The model under review builds one solid part; all positions refer to its coordinate system, in mm. Face numbers are marked on the shaded views. A direction names the side the tool comes from. Round coordinates to 2 decimals unless told otherwise and drop trailing zeros. Order: outer loops, then holes, each group sorted by start corner. A loop starts at its lowest first (then second) coordinate and runs counter-clockwise, first axis right, second up. Notation, with made-up numbers: M -26,72 L 10,72 A21 ccw 10,76 Z; hole C 76.5,56 d5. An arc over 180 degrees is marked long. Answer as a JSON object with one key per item and string values. Group by question number.
1. Add section C-C on y = 0.25. State the section outline as (x, z) points.
2. Add section A-A on z = 4.5. State the section outline as (x, y) points.
3. To check wall thickness, follow probe 1 along Y at (x, z) = (-1, -2.5); probe 2 along Y at (x, z) = (-1.5, 6.5); probe 3 along Z at (x, y) = (-2.25, 3). State the ranges of each line that lie inside material, in increasing order. Write a range as [from, to].
4. Add section D-D on z = -5.75. State the section outline as (x, y) points, and give its area (4 significant figures).
5. Mouldability with a two-part tool opening along Y and no side actions: class the marked faces 1, 2, 3 and 4 as released by +Y, released by -Y, zero draft, split by the parting line, or undercut.
6. Clearance check with flat-ended pins moving along their axes: P1, Ø0.5, axis at y = -0.5, z = -4.5, coming from the +X side; P2, Ø3, axis at x = 0, z = 0, coming from the +Y side. State where each tip first meets the part, or that it passes through.
7. Machinability: for the marked faces 5 and 6, which of the approach directions +Z, -Z, +X, -X, +Y, -Y give a long, thin tool a straight path to every point of the face, cutting with its end or side? Answer none if there is none.
8. Add section B-B on x = -0.25. State the section outline as (y, z) points, and give its area (3 significant figures).
Autodesk Inventor part; units mm, degrees
ref_plane "YZ Plane" through (0, 0, 0) normal (1, 0, 0) x (0, 1, 0)
ref_plane "XZ Plane" through (0, 0, 0) normal (0, 1, 0) x (-1, 0, 0)
ref_plane "XY Plane" through (0, 0, 0) normal (0, 0, 1) x (1, 0, 0)
sketch "スケッチ1" plane through (0, 0, 0) normal (0, 1, 0) x (-1, 0, 0)
  circle A0 centre (0, 0) radius 1.15
  circle A1 centre (0, 0) radius 2
  circle A2 centre (0, 0) radius 3.5
  line L0 (0, 0) -> (0, 3.5)
  line L1 (2, 0) -> (-2, 0)
  line L2 (2, 0) -> (2, -2.8723)
  line L3 (-2, 0) -> (-2, -2.8723)
  line L4 (0, 2) -> (3.5, 2)
  line L5 (3.5, 2) -> (3.5, 6)
  line L6 (3.5, 6) -> (0, 6)
  line L7 (0, 6) -> (0, 2)
  line L8 (0, 6) -> (3.5, 6)
  line L9 (3.5, 6) -> (3.5, 0)
  line L10 (3.5, 0) -> (0, 0)
  line L11 (0, 0) -> (0, 6)
  line L12 (0, 0) -> (0, -8)
  line L13 (0, 0) -> (3.5, 0)
  line L14 (3.5, 0) -> (3.5, -8)
  line L15 (3.5, -8) -> (0, -8)
  line L16 (0, -8) -> (0, 0)
  line L17 (2, -2.8723) -> (2, -8)
  line L18 (0, -8) -> (3.5, -4.5)
  line L19 (0, -8) -> (4.9497, -8) construction
  line L20 (0, 0) -> (3.5, 0)
  line L21 (3.5, 0) -> (3.5, -9)
  line L22 (3.5, -9) -> (0, -9)
  line L23 (0, -9) -> (0, 0)
  line L24 (0, 2) -> (4, 2)
  line L25 (4, 2) -> (4, 9)
  line L26 (4, 9) -> (0, 9)
  line L27 (0, 9) -> (0, 2)
  line L28 (0, 9) -> (4, 9)
  line L29 (4, 9) -> (4, -9)
  line L30 (4, -9) -> (0, -9)
  line L31 (0, -9) -> (0, 9)
  line L32 (0, 0) -> (2, 0)
  line L33 (2, 0) -> (2, -9)
  line L34 (2, -9) -> (0, -9)
  line L35 (0, -9) -> (0, 0)
  point P0 (2, -6)
  point P1 (0, -3.5)
  dimension "d0" = 2.3
  dimension "d1" = 4
  dimension "d2" = 7
  dimension "d3" = 3.5
  dimension "d4" = 4
  dimension "d5" = 8
  dimension "d6" = 45
  dimension "d40" = 9
  dimension "d41" = 4
  dimension "d42" = 7
extrude "押し出し1" add sketch "スケッチ1" along normal blind 3 contours A1 L3 A2 L0
extrude "押し出し2" add sketch "スケッチ1" along normal blind 4.5 contours L10 A2 L2 | A1 L4 A2 L10 | L0 A2 L4 | A2 L14 L18 L17 | A2 L4 L9 | L9 L24 L29 L30 L21 L14 | L7 L6 L5 L4 A2 | L18 L14 L15 L17 | L5 L6 L27 L26 L25 L24 | L15 L21 L22 L33
extrude "押し出し3" add sketch "スケッチ1" against normal blind 1 contours L1 A1 L12 A0 | A0 L0 A1 L1 | A0 L1 A1 L0 | L12 A1 L1 A0 | L2 A2 L12 A1 | L10 A2 L2 | A1 L4 A2 L10 | A1 L3 A2 L0 | L0 A2 L4 | L12 A2 L3 A1 | L17 L18 L12 A2 | A2 L14 L18 L17 | A2 L4 L9 | L9 L24 L29 L30 L21 L14 | L7 L6 L5 L4 A2 | L18 L14 L15 L17 | L17 L15 L18 | L5 L6 L27 L26 L25 L24 | L15 L33 L22 L23 | L15 L21 L22 L33
sketch "スケッチ4" plane through (0, 4.5, 0) normal (0, 1, 0) x (1, 0, 0)
  circle A0 centre (0, 0) radius 1.15
  circle A1 centre (0, 0) radius 2
  circle A2 centre (0, 0) radius 3.5
  line L0 (-4, 9) -> (-4, -9)
  line L1 (0, 0) -> (-4, 0)
  line L2 (-4, 0) -> (-4, -9)
  line L3 (-4, -9) -> (0, -9)
  line L4 (0, -9) -> (0, 0)
  line L5 (0, 0) -> (-4, 0)
  line L6 (-4, 0) -> (-4, 9)
  line L7 (-4, 9) -> (0, 9)
  line L8 (0, 9) -> (0, 0)
  point P0 (0, -3.5)
  point P1 (0, 3.5)
  dimension "d43" = 2.3
  dimension "d44" = 4
  dimension "d45" = 7
  dimension "d46" = 4
  dimension "d47" = 9
extrude "押し出し6" add sketch "スケッチ4" along normal blind 1 contours A0 L8 A1 L4 | A0 L1 A1 L8 | L4 A1 L1 A0 | L8 A2 L4 A1 | A1 L1 A2 L8 | L4 A2 L1 A1 | A2 L1 L0 L7 L8 | L4 L3 L0 L1 A2
sketch "スケッチ5" plane through (-4, -1, 9) normal (0, 0, 1) x (1, 0, 0)
  line L0 (4, 0) -> (4, 4)
  line L1 (4, 0) -> (0, 0)
  line L2 (0, 0) -> (0, 1)
  line L3 (0, 1) -> (4, 1)
  line L4 (4, 1) -> (4, 0)
  line L5 (4, 1) -> (2.5, 1)
  line L6 (2.5, 1) -> (2.5, 1.5)
  line L7 (2.5, 1.5) -> (4, 1.5)
  line L8 (4, 1.5) -> (4, 1)
  line L9 (4, 6.5) -> (0, 6.5)
  line L10 (0, 6.5) -> (2, 6.5)
  line L11 (2, 6.5) -> (2, 4.25)
  line L12 (2, 4.25) -> (0, 4.25)
  line L13 (0, 4.25) -> (0, 6.5)
  circle A0 centre (2, 4.25) radius 1.1
  dimension "d50" = 4
  dimension "d51" = 1
  dimension "d52" = 1.5
  dimension "d53" = 0.5
  dimension "d54" = 2
  dimension "d55" = 2.25
  dimension "d56" = 2.2
extrude "押し出し7" cut sketch "スケッチ5" against normal blind 7 contours A0 L12 L11 | L11 L12 A0
hole "穴2" at (-1.5, 0.5, 9) direction (0, 0, -1) diameter 1 end through all
chamfer "面取り1" distance 0.5 angle 45 3 edges at (0, -1, 6.25) (0, 5.5, 6.25) (-4, 5.5, 0)
chamfer "面取り2" distance 1.5 angle 45 1 edges at (-4, -1, 0)
sketch "スケッチ6" plane through (0, 0, -9) normal (0, 0, -1) x (-1, 0, 0)
  line L0 (0, 5.5) -> (4, 5.5)
  line L1 (4, 5.5) -> (4, -1)
  line L2 (4, -1) -> (0, -1)
  line L3 (0, -1) -> (0, 5.5)
  point P0 (0, 0)
  dimension "d72" = 4
  dimension "d73" = 6.5
extrude "押し出し8" cut sketch "スケッチ6" against normal blind 1
chamfer "面取り3" distance 0.2 angle 45 2 edges at (-1.75, 5.5, -8) (-1.25, -1, -8)
properties part number "rod6.3"
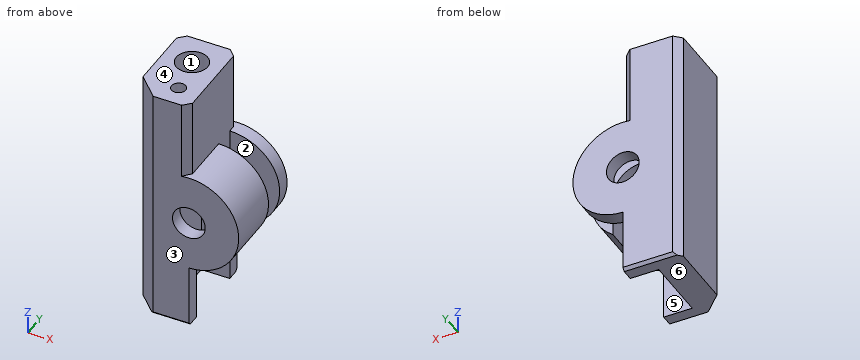
Recorded:
{
 "1": {"outline": "M -3.75,-8 L -2,-8 L -2,0 A2 cw -1.93,0.51 L -1.93,9 L -3.75,9 Z; M -1.07,1.69 A2 cw 2,0 L 2,-2.87 A3.5 ccw 0,3.5 L 0,9 L -1.07,9 Z"},
 "2": {"outline": "M -4,0.5 L -2.5,-1 L -0.5,-1 L 0,-0.5 L 0,5 L -0.5,5.5 L -3.5,5.5 L -4,5 Z; hole C -2,3.25 d2.2; hole C -1.5,0.5 d1"},
 "3": {"probe 1": "y = [-1, 0], [4.5, 5.5]", "probe 2": "y = [-1, 0], [1, 2.27], [4.23, 5.5]", "probe 3": "z = [-8, 2]"},
 "4": {"outline": "M -4,0.5 L -2.5,-1 L 0,-1 L 0,0 L -2,0 L -2,4.5 L 0,4.5 L 0,5.5 L -3.5,5.5 L -4,5 Z", "area": "15.75 mm²"},
 "5": {"face 1": "undercut", "face 2": "undercut", "face 3": "released by -Y", "face 4": "zero draft"},
 "6": {"P1": "stops at x = 0", "P2": "stops at y = 5.5"},
 "7": {"face 5": "-Z", "face 6": "-Z, +X, -X, +Y, -Y"},
 "8": {"outline": "M -1,-7.8 L -0.8,-8 L 0,-8 L 0,-1.12 L -1,-1.12 Z; M -1,1.12 L 0,1.12 L 0,1.98 L 4.5,1.98 L 4.5,1.12 L 5.5,1.12 L 5.5,3.49 L 5.25,3.49 L 5.25,9 L -0.75,9 L -0.75,3.49 L -1,3.49 Z; M 4.5,-8 L 5.3,-8 L 5.5,-7.8 L 5.5,-1.12 L 4.5,-1.12 Z", "area": "58.3 mm²"}
}
